Input: part model. Units: mm. Frame: model coordinates. A direction names the side the tool comes from. Round coordinates to 2 decimals unless told otherwise and drop trailing zeros. Order: outer loops, then holes, each group sorted by start corner. A loop starts at its lowest first (then second) coordinate and runs counter-clockwise, first axis right, second up. Notation, with made-up numbers: (-13.5, 33.5) -> (16.5, 33.5) arc R15 ccw to (16.5, 39.5) -> close; hole circle Ø10 at (29, 56.5). An arc over 180 degrees is marked (long way). Answer as CSV lines item,"result". Start each with the question number.
1) Section query B-B, the plane z = -19. Output: boundary loops of the cut face in (x, y), and give its area (3 significant figures).
2) Mould query, pull axis Z, two halves, no side actions, for faces 3 (the face through (-7, 2.6, -20)), 4 (the face through (5.4, 6, 20)), 5 (the face through (0, 5, -23)), 6 (the face through (10, 5, 0)). Classes: +Z half, -Z half, draft (parallel to the pull), parting line (faces both ways), or undercut.
3) Section query C-C, the plane x = 0. Output: boundary loops of the cut face in (y, z).
4) First-contact query: P1, Ø2, axis at x = -0.5, z = 11, coming from the +Y side; P2, Ø0.9, axis at x = -6.5, z = -20, coming from the +Y side. Flat tips, straight axial feed; report the tip coordinate or a pass-through.
5) Access query for faces 1 (the face through (7, 2.6, -20)), 2 (the face through (8.5, 2, 0)). Directions: +Z, -Z, +X, -X, +Y, -Y. A direction counts if a zero-diameter tool reaches every point of the face in a straight line with its end or side. Return the directions, or none.
6) Section query A-A, the plane y = 1.5. Output: boundary loops of the cut face in (x, z), and give its area (3 significant figures).
7) Section query D-D, the plane z = 16.5. Output: boundary loops of the cut face in (x, y).
8) Line query: L1, parallel to Z at x = 7.25, y = 6.5; L2, parallel to X at y = 8.75, z = 20.5; L3, parallel to X at y = 4.45, z = 11.5. Output: solid intervals per line, ascending.
```python
from build123d import *

# Parameters (mm, degrees)
SKETCH1_W           = 20
SKETCH1_H           = 42
BOSS_EXTRUDE1_DEPTH = 7.6
CUT_EXTRUDE1_DEPTH  = 4
THICKEN1_START      = -10
THICKEN1_DEPTH      = 20
SKETCH3_R           = 3.25
CUT_EXTRUDE2_DEPTH  = 1.6
SKETCH5_W           = 3
SKETCH5_H           = 3
CUT_EXTRUDE4_DEPTH  = 7
SKETCH6_W           = 14
SKETCH6_H           = 31.6
CUT_EXTRUDE5_DEPTH  = 3


# Read off the part's stored shape, not the designer's step: Thicken1
with BuildPart() as part:
    # Sketch1 → Boss-Extrude1 (new body)
    with BuildSketch(Plane(origin=(0, 0, 0), x_dir=(1, 0, 0), z_dir=(0, 1, 0))):
        Rectangle(SKETCH1_W, SKETCH1_H)
    extrude(amount=BOSS_EXTRUDE1_DEPTH)

    # Sketch2 → Cut-Extrude1 (cut)
    with BuildSketch(Plane.XZ):
        with BuildLine():
            Line((5.5, 2), (8.5, 2))
            Line((8.5, 2), (8.5, -2))
            Line((8.5, -2), (5.5, -2))
            ThreePointArc((5.5, -2), (4.085786438, -2.585786438), (3.5, -4))
            Line((3.5, -4), (3.5, -17.5))
            Line((3.5, -17.5), (-3.5, -17.5))
            Line((-3.5, -17.5), (-3.5, -4))
            ThreePointArc((-3.5, -4), (-4.085786438, -2.585786438), (-5.5, -2))
            Line((-5.5, -2), (-8.5, -2))
            Line((-8.5, -2), (-8.5, 2))
            Line((-8.5, 2), (-5.5, 2))
            ThreePointArc((-5.5, 2), (-4.085786438, 2.585786438), (-3.5, 4))
            Line((-3.5, 4), (-3.5, 17.5))
            Line((-3.5, 17.5), (3.5, 17.5))
            Line((3.5, 17.5), (3.5, 4))
            ThreePointArc((3.5, 4), (4.085786438, 2.585786438), (5.5, 2))
        make_face()
    extrude(amount=-CUT_EXTRUDE1_DEPTH, mode=Mode.SUBTRACT)

    # Thicken1 outline → Thicken1 (add)
    with BuildSketch(Plane.YZ.offset(THICKEN1_START)):
        Polygon((0, -23), (9.6, -23), (9.6, 23), (0, 23), (0, 21), (7.6, 21), (7.6, -21), (0, -21), align=None)
    extrude(amount=THICKEN1_DEPTH)

    # Sketch3 → Cut-Extrude2 (cut)
    with BuildSketch(Plane.XZ.offset(-4)):
        with Locations(Location((0, 11.5, 0), (0, 0, 270))):
            Circle(SKETCH3_R)
        with Locations(Location((0, -11.5, 0), (0, 0, 90))):
            Circle(SKETCH3_R)
    extrude(amount=-CUT_EXTRUDE2_DEPTH, mode=Mode.SUBTRACT)

    # Sketch5 → Cut-Extrude4 (cut)
    with BuildSketch(Plane(origin=(0, 9.6, 0), x_dir=(1, 0, 0), z_dir=(0, 1, 0))):
        with Locations((-6.9, 19.9)):
            Rectangle(SKETCH5_W, SKETCH5_H)
        with Locations((6.9, 19.9)):
            Rectangle(SKETCH5_W, SKETCH5_H)
        with Locations((6.9, -19.9)):
            Rectangle(SKETCH5_W, SKETCH5_H)
        with Locations((-6.9, -19.9)):
            Rectangle(SKETCH5_W, SKETCH5_H)
    extrude(amount=-CUT_EXTRUDE4_DEPTH, mode=Mode.SUBTRACT)

    # Sketch6 → Cut-Extrude5 (cut)
    with BuildSketch(Plane(origin=(0, 9.6, 0), x_dir=(1, 0, 0), z_dir=(0, 1, 0))):
        Rectangle(SKETCH6_W, SKETCH6_H)
    extrude(amount=-CUT_EXTRUDE5_DEPTH, mode=Mode.SUBTRACT)


solid = part.part
```
Findings:
1,outline,"(-10, 0) -> (10, 0) -> (10, 9.6) -> (8.4, 9.6) -> (8.4, 2.6) -> (5.4, 2.6) -> (5.4, 9.6) -> (-5.4, 9.6) -> (-5.4, 2.6) -> (-8.4, 2.6) -> (-8.4, 9.6) -> (-10, 9.6) -> close"
1,area,"150 mm^2"
2,face 3,"undercut"
2,face 4,"undercut"
2,face 5,"-Z half"
2,face 6,"draft"
3,outline,"(0, -23) -> (9.6, -23) -> (9.6, -15.8) -> (6.6, -15.8) -> (6.6, 15.8) -> (9.6, 15.8) -> (9.6, 23) -> (0, 23) -> (0, 17.5) -> (4, 17.5) -> (4, 14.75) -> (5.6, 14.75) -> (5.6, 8.25) -> (4, 8.25) -> (4, -8.25) -> (5.6, -8.25) -> (5.6, -14.75) -> (4, -14.75) -> (4, -17.5) -> (0, -17.5) -> close"
4,P1,"stops at y = 6.6"
4,P2,"stops at y = 2.6"
5,face 1,"+Y"
5,face 2,"-Y"
6,outline,"(-10, -23) -> (10, -23) -> (10, 23) -> (-10, 23) -> close; hole (-8.5, -2) -> (-5.5, -2) arc R2 cw to (-3.5, -4) -> (-3.5, -17.5) -> (3.5, -17.5) -> (3.5, -4) arc R2 cw to (5.5, -2) -> (8.5, -2) -> (8.5, 2) -> (5.5, 2) arc R2 cw to (3.5, 4) -> (3.5, 17.5) -> (-3.5, 17.5) -> (-3.5, 4) arc R2 cw to (-5.5, 2) -> (-8.5, 2) -> close"
6,area,"632 mm^2"
7,outline,"(-10, 0) -> (-3.5, 0) -> (-3.5, 4) -> (3.5, 4) -> (3.5, 0) -> (10, 0) -> (10, 9.6) -> (-10, 9.6) -> close"
8,L1,"z = -23 to -21.4, -18.4 to 18.4, 21.4 to 23"
8,L2,"x = -10 to -8.4, -5.4 to 5.4, 8.4 to 10"
8,L3,"x = -10 to -3.25, 3.25 to 10"
